Can you work these out from the model? Positions are in its coordinate system, mm. A direction names the side the tool comes from. Round coordinates to 2 decimals unless told otherwise and drop trailing zeros. Write each loop counter-clockwise with the first axis right and the second up, starting at its lowest first coordinate (ties: lowest second). Pieces come first, ordered by that corner, then holes. Notation, with made-up numbers: (16, 20) -> (24, 20) arc R28 ccw to (24, 46) -> close; hole circle Ø6 at (22, -29). An arc over 180 degrees is marked (long way). Write item = value, one per line. Start each with the question number.
1) Imagine slicing it at A-A, the plane x = 0. State how many separate pieces and enclosed holes the cut face has, then the cut area to 3 significant figures.
2) I'm going to push flat-ended pins straight in: pin 1 (4 mm diameter, centred on y = 11.5, z = 2, fed in from -X); pin 2 (1.9 mm diameter, centred on y = 0.5, z = 0, fed in from +X); pin 3 (3 mm diameter, centred on x = 0, y = 2, fed in from -Z). Where does each tip first touch, or does it pass through?
3) For faces 1 (the face through (8.731, -1, 3)), 2 (the face through (0, 0, 13)), which set-ups out of +Z, -Z, +X, -X, +Y, -Y let a thin tool reach every point of the face, with its end or its side?
4) Thinking about a two-plate mould opening in X: for faces 3 (the face through (11.126, 4.785, 0.207)), 4 (the face through (0.61, -1.61, 11.47)), 5 (the face through (0, -3.175, 5)), 6 (the face through (-0.19, -1.57, 17.46)), which applies, +X half, -X half, draft (parallel to the pull), parting line (faces both ways), or undercut?
5) Imagine slicing it at B-B, the plane y = 5.75. Please give me the cut outline in (x, z) (1 decimal), then the cut area to 3 significant figures.
6) If I drill on line 1 (Y direction, x = 2, z = 15.5) (3 decimals); line 2 (X direction, y = 3.5, z = 0.75); line 3 (Y direction, x = -2, z = 2.75) (3 decimals), over which ranges is the centre line in solid material (lowest first)?
from build123d import *

# Parameters (mm, degrees)
SKETCH3_R                  = 1.5875
SKETCH4_R                  = 1.5875
BOSS_EXTRUDE1_DEPTH        = 8.73125
FILLET1_RADIUS             = 8.73125
FILLET1_LENGTH             = 3.175
F_2_0_221_DIAMETER_HOLE1_D = 5.6134


with BuildPart() as part:
    # Sweep1: sweep along a path in Sketch2
    with BuildLine(Plane.XY) as sweep1_path:
        Line((-9.525, 0), (9.525, 0))
        ThreePointArc((9.525, 0), (11.77006403, 0.92993597), (12.7, 3.175))
        Line((12.7, 3.175), (12.7, 6.35))
        ThreePointArc((12.7, 6.35), (0, 19.05), (-12.7, 6.35))
        Line((-12.7, 6.35), (-12.7, 3.175))
        ThreePointArc((-12.7, 3.175), (-11.77006403, 0.92993597), (-9.525, 0))
    # Sketch3 → Sweep1 (sweep)
    with BuildSketch(Plane(origin=(0, 0, 0), x_dir=(0, 0, -1), z_dir=(1, 0, 0))):
        Circle(SKETCH3_R)
    sweep(path=sweep1_path.line)

    # Sketch4 → Boss-Extrude1 (add, symmetric)
    with BuildSketch(Plane(origin=(0, 0, 0), x_dir=(0, 0, -1), z_dir=(1, 0, 0))):
        with BuildLine():
            Line((-17.4625, -3.175), (0, -3.175))
            ThreePointArc((0, -3.175), (2.749630657, 1.5875), (-2.749630657, 1.5875))
            ThreePointArc((-2.749630657, 1.5875), (-3.911761314, 0.425369343), (-5.499261314, 0))
            Line((-5.499261314, 0), (-17.4625, 0))
            Line((-17.4625, 0), (-17.4625, -3.175))
        make_face()
        with Locations(Location((0, 0, 0), (0, 0, 180))):
            Circle(SKETCH4_R, mode=Mode.SUBTRACT)
    extrude(amount=BOSS_EXTRUDE1_DEPTH, both=True)

    # Fillet1: full round fillet: the end face becomes a half cylinder, R = half its width
    fillet1_face = Plane((0, -1.5875, 17.4625), x_dir=(0, 1, 0), z_dir=(0, 0, 1))  # on the end face: x along it, z out of the body
    fillet1_slab = fillet1_face.offset(-FILLET1_RADIUS / 2) * Box(FILLET1_LENGTH, 2 * FILLET1_RADIUS, FILLET1_RADIUS, mode=Mode.PRIVATE)  # the body's end, R deep
    fillet1_round = Plane((0, -1.5875, 8.73125), x_dir=(0, 0, 1), z_dir=(0, 1, 0)) * Cylinder(FILLET1_RADIUS, FILLET1_LENGTH, mode=Mode.PRIVATE)  # its axis R under the face
    add(fillet1_slab - fillet1_round, mode=Mode.SUBTRACT)

    # #2 (0.221) Diameter Hole1 (through all)
    with Locations(Plane(origin=(0, 0, 0), x_dir=(1, 0, 0), z_dir=(0, 1, 0))):
        with Locations((0, -8.73125)):
            Hole(F_2_0_221_DIAMETER_HOLE1_D / 2)


solid = part.part
Reported:
q1.separate_pieces = 3
q1.enclosed_holes = 0
q1.area = 70.1 mm²
q2.pin_1 = -13.68
q2.pin_2 = 13.96
q2.pin_3 = -3.14
q3.face_1 = none
q3.face_2 = +Z, +X, -X, +Y
q4.face_3 = undercut
q4.face_4 = undercut
q4.face_5 = draft
q4.face_6 = parting line
q5.outline = circle Ø3.2 at (-12.7, 0); circle Ø3.2 at (12.7, 0)
q5.area = 15.8 mm²
q6.line_1 = -3.175 to 0
q6.line_2 = -14.1 to -11.3, 11.3 to 14.1
q6.line_3 = -3.175 to 1.587
